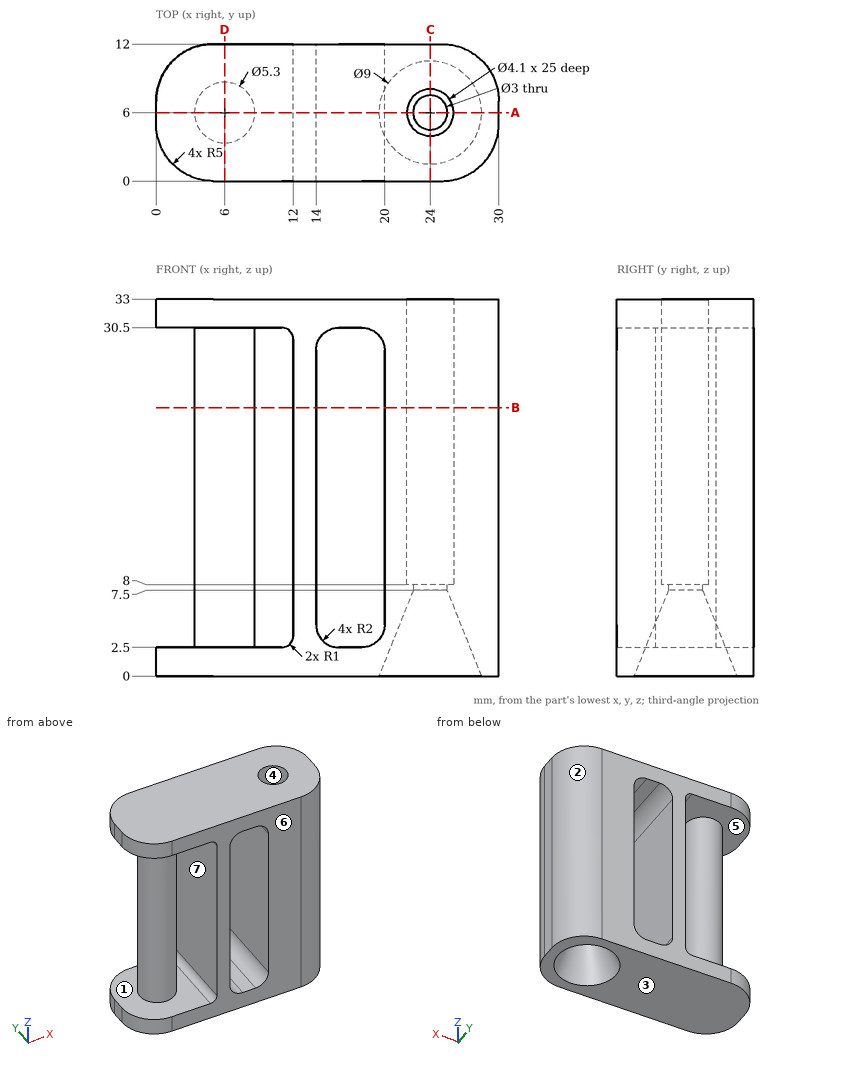
Drawing for the job (mm, zero at the part's lowest x, y, z). A direction names the side the tool comes from. Give positions to 0.01 mm unless a question says otherwise; leave off trailing zeros. Write each loop counter-clockwise with the first axis right and the second up, starting at its lowest first coordinate (ties: lowest second). Pieces come first, ordered by that corner, then holes. Notation, with made-up numbers: (-15, 14.25) -> (-7, 14.25) arc R29 ccw to (-7, 52.25) -> close; hole circle Ø1 at (60.25, -1.75). An arc over 180 degrees is marked (long way). Put each result on its own line as item: value. Start each with the question number.
Item 1: Wall check: L1, parallel to Z at x = 17, y = 4.75; L2, parallel to X at y = 7.25, z = 4; L3, parallel to Y at x = 24, z = 11. Give the ranges that are in metal, low to high. Write a range as [from, to].
Item 2: Cut at B-B (z = 23.5). List the corners of the cut face in (x, y).
Item 3: Cut at D-D (x = 6). List the corners of the cut face in (y, z).
Item 4: Cut at A-A (y = 6). State how many separate pieces and enclosed holes the cut face has, then the cut area to 3 significant figures.
Item 5: Pull direction Z, two halves, no side cores. Call the marked faces 1, 2 and 3: pulls with the +Z half, pulls with the -Z half, needs draft (parallel to the pull), parting line crosses it, or undercut.
Item 6: Pin check, flat tips, straight feed: pin 1 Ø1.5 at (x, z) = (26, 20.5) entering from +Y; pin 2 Ø1.5 at (x, y) = (22, 5) entering from -Z; pin 3 Ø1.5 at (x, z) = (4, 23) entering from +Y; pin 4 Ø1.8 at (x, y) = (24, 6) entering from +Z. Stop position of each tip, or through.
Item 7: Which spindle directions (+Z, -Z, +X, -X, +Y, -Y) get a long thin tool onto all of the face, cutting with end or side? Do the marked faces 4, 5, 6 and 7. Say none if no direction does.
Item 8: Cut at C-C (x = 24). List the corners of the cut face in (y, z).
Answer list:
1. L1: z = [0, 2.5], [30.5, 33]
1. L2: x = [3.66, 8.34], [12, 14.06], [19.94, 21.38], [26.62, 29.99]
1. L3: y = [0, 3.95], [8.05, 12]
2. outline: circle Ø5.3 at (6, 6); (12, 0) -> (14, 0) -> (14, 12) -> (12, 12) -> close; (20, 0) -> (25, 0) arc R5 ccw to (30, 5) -> (30, 7) arc R5 ccw to (25, 12) -> (20, 12) -> close; hole circle Ø4.1 at (24, 6)
3. outline: (0, 0) -> (12, 0) -> (12, 2.5) -> (8.65, 2.5) -> (8.65, 30.5) -> (12, 30.5) -> (12, 33) -> (0, 33) -> (0, 30.5) -> (3.35, 30.5) -> (3.35, 2.5) -> (0, 2.5) -> close
4. separate pieces: 2
4. enclosed holes: 2
4. area: 489 mm2
5. face 1: undercut
5. face 2: needs draft
5. face 3: pulls with the -Z half
6. pin 1: stops at y = 11.99
6. pin 2: stops at z = 3.78
6. pin 3: stops at y = 8.34
6. pin 4: passes through
7. face 4: +Z
7. face 5: none
7. face 6: +Z, -Z, +X, -X, -Y
7. face 7: +Y, -Y
8. outline: (0, 0) -> (1.5, 0) -> (4.5, 7.5) -> (4.5, 8) -> (3.95, 8) -> (3.95, 33) -> (0, 33) -> close; (7.5, 7.5) -> (10.5, 0) -> (12, 0) -> (12, 33) -> (8.05, 33) -> (8.05, 8) -> (7.5, 8) -> close
